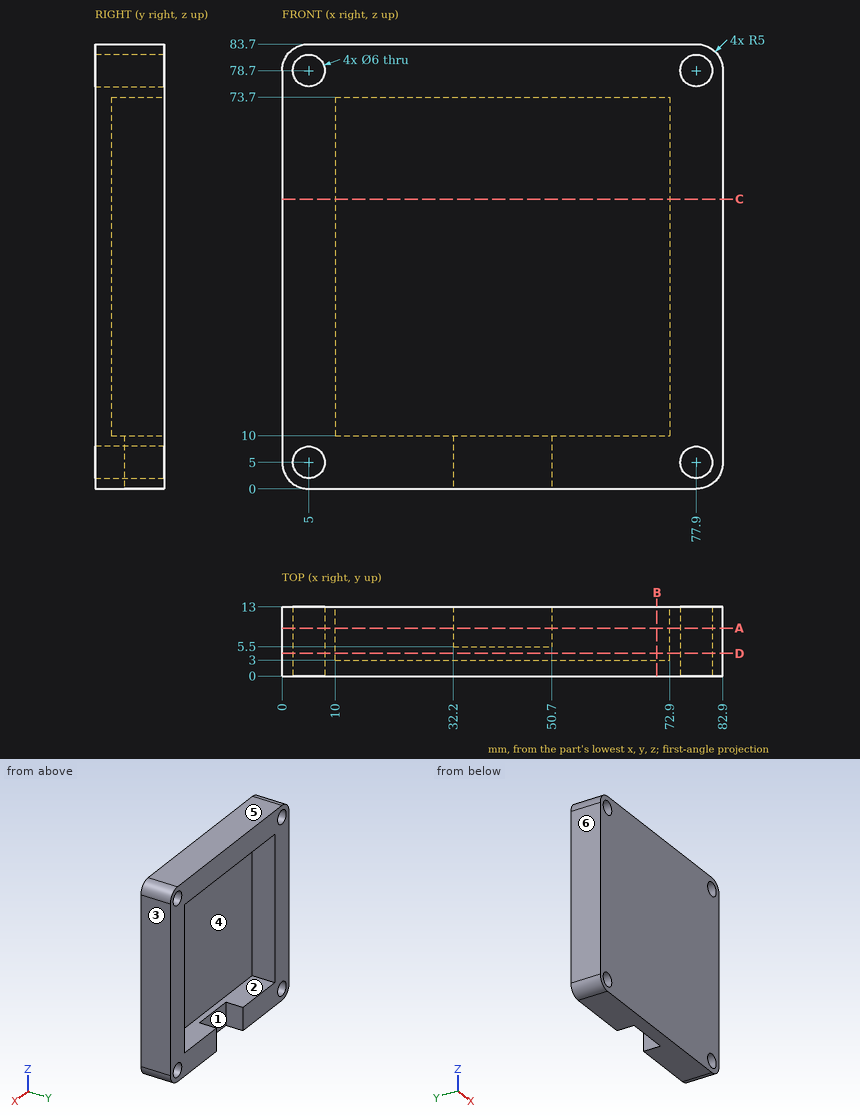
Drawing for the job (mm, zero at the part's lowest x, y, z). A direction names the side the tool comes from. Give positions to 0.01 mm unless a question says otherwise; leave off trailing zeros. Write each loop counter-clockwise with the first axis right and the second up, starting at its lowest first coordinate (ties: lowest second). Pieces come first, ordered by that corner, then holes. Notation, with made-up numbers: M 26,-1 L 76,-1 A19 ccw 76,22 Z; hole C -27,33.5 d5. An arc over 180 degrees is marked long. Return JSON: item names as keys, results as strings. Group by question number.
(1) Band-saw the part on B-B (x = 70.5). Give the cut face in (y, z).
(2) 3-axis set-ups, long thin cutter, end or side, ignore diameter. For the marked faces 1, 2 and 3: which of +Z, -Z, +X, -X, +Y, -Y reach the whole face in a straight line?
(3) Flat gauge pins, fed straight in: pin 1 Ø1 at (x, y) = (47.5, 10) entering from -Z; pin 2 Ø5 at (x, z) = (5, 5) entering from -Y; pin 3 Ø2 at (x, z) = (42.5, 14.5) entering from +Y; pin 4 Ø8 at (x, z) = (45, 7.5) entering from +Y. Where does each tip first touch, or does it go through?
(4) Mould opens along X. For the marked faces 4, 5 and 6 say: pulls with the +X half, pulls with the -X half, needs draft (parallel to the pull), parting line crosses it, or undercut.
(5) Band-saw the part on C-C (z = 54.5). Give the cut face in (x, y).
(6) Band-saw the part on A-A (y = 9). Give the cut face in (x, z), and give its area (3 significant figures).
(7) Drill centre lines: L1, parallel to X at y = 5, z = 5; L2, parallel to Z at x = 77.9, y = 8.5; L3, parallel to Z at x = 11, y = 9. Where is each one in solid material? Low to high. Write a range as [from, to].
(8) Band-saw the part on D-D (y = 4.25). Give the cut face in (x, z).
Entries:
{
 "1": {"outline": "M 0,0 L 13,0 L 13,10 L 3,10 L 3,73.7 L 13,73.7 L 13,83.7 L 0,83.7 Z"},
 "2": {"face 1": "-Z, +Y", "face 2": "+Y", "face 3": "+Z, -Z, +X, +Y, -Y"},
 "3": {"pin 1": "stops at z = 73.7", "pin 2": "passes through", "pin 3": "stops at y = 3", "pin 4": "stops at y = 5.5"},
 "4": {"face 4": "undercut", "face 5": "needs draft", "face 6": "pulls with the -X half"},
 "5": {"outline": "M 0,0 L 82.9,0 L 82.9,13 L 72.9,13 L 72.9,3 L 10,3 L 10,13 L 0,13 Z"},
 "6": {"outline": "M 0,5 A5 ccw 5,0 L 32.2,0 L 32.2,10 L 10,10 L 10,73.7 L 72.9,73.7 L 72.9,10 L 50.7,10 L 50.7,0 L 77.9,0 A5 ccw 82.9,5 L 82.9,78.7 A5 ccw 77.9,83.7 L 5,83.7 A5 ccw 0,78.7 Z; hole C 5,5 d6; hole C 5,78.7 d6; hole C 77.9,5 d6; hole C 77.9,78.7 d6", "area": "2,610 mm^2"},
 "7": {"L1": "x = [0, 2], [8, 74.9], [80.9, 82.9]", "L2": "z = [0, 2], [8, 75.7], [81.7, 83.7]", "L3": "z = [0, 10], [73.7, 83.7]"},
 "8": {"outline": "M 0,5 A5 ccw 5,0 L 77.9,0 A5 ccw 82.9,5 L 82.9,78.7 A5 ccw 77.9,83.7 L 5,83.7 A5 ccw 0,78.7 Z; hole C 5,5 d6; hole C 5,78.7 d6; hole M 10,10 L 72.9,10 L 72.9,73.7 L 10,73.7 Z; hole C 77.9,5 d6; hole C 77.9,78.7 d6"}
}
